from build123d import *

# Parameters (mm, degrees)
F0_R     = 18.85
F0_R_2   = 3.625
F1_DEPTH = 8
F2_SIZE  = 2
F3_T     = -1.5


with BuildPart() as f1:
    # F0 (on Top) → F1 (new body)
    with BuildSketch(Plane.XY):
        Circle(F0_R)
        Circle(F0_R_2, mode=Mode.SUBTRACT)
    extrude(amount=F1_DEPTH)

    # F2
    f2_edges = [f1.edges().sort_by_distance(p)[0] for p in [
        (-18.85, 0, 8),
    ]]
    chamfer(f2_edges, length=F2_SIZE)

    # F3
    f3_openings = [f1.faces().sort_by_distance(p)[0] for p in [
        (-18.316841, 0, 0),
    ]]
    offset(amount=F3_T, openings=f3_openings)


solid = f1.part
Input: part model. Units: mm. Frame: model coordinates. A direction names the side the tool comes from. Round coordinates to 2 decimals unless told otherwise and drop trailing zeros. Loops run counter-clockwise (first coordinate to the right, second up) from the corner with the lowest first, then second, coordinate; pieces in that order, holes last. Notation, with made-up numbers: M -17.5,74.5 L -6.5,74.5 A35 cw -6.5,111.5 Z; hole C 61,-4.5 d4. An arc over 180 degrees is marked long. Answer as CSV lines item,"result". Start each with the question number.
(1) First-contact query: pin 1 (8 mm diameter, centred on x = -7, y = 11, fed in from -Z); pin 2 (1.5 mm diameter, centred on x = -10.5, z = 7, fed in from +Y); pin 3 (3 mm diameter, centred on x = -8.5, z = 6, fed in from -Y). Flat tips, straight axial feed; report the tip coordinate or a pass-through.
(2) Draft query along Y for faces 1 (the flat face through (2.2, -3.3, 0)), 2 (the cylindrical face through (-1.111, -5.003, 3.204)), 3 (the cylindrical face through (-4.1, -18.4, 3)). Return one class per face: released by +Y, released by -Y, zero draft, split by the parting line, or undercut.
(3) Reachability of faces 4 (the flat face through (17, -5, 0)), 5 (the flat face through (-4, 4, 6.5)) from +Z, -Z, +X, -X, +Y, -Y: full face, straight path, thin tool, end or side. Return the list, or none.
(4) Section A-A, the plane y = 0. Output: boundary loops of the cut face in (x, z) (3 decimals), plus the area to 3 significant figures.
(5) Section C-C, the plane z = 2.25. Output: boundary loops of the cut face in (x, y) (3 decimals), plus the area to 3 significant figures.
(6) Line query: line 1 (Y direction, x = 0, z = 2) (3 decimals); line 2 (Z direction, x = 13, y = 1.5); line 3 (Y direction, x = 0, z = 5.75) (3 decimals). Output: solid intervals per line, ascending. Write a range as [from, to].
Values found:
1,pin 1,"stops at z = 5.69"
1,pin 2,"stops at y = 15.48"
1,pin 3,"stops at y = -17.5"
2,face 1,"zero draft"
2,face 2,"undercut"
2,face 3,"split by the parting line"
3,face 4,"-Z, +X, -X, +Y, -Y"
3,face 5,"-Z"
4,outline,"M -18.85,0 L -17.35,0 L -17.35,5.379 L -16.229,6.5 L -5.125,6.5 L -5.125,0 L -3.625,0 L -3.625,8 L -16.85,8 L -18.85,6 Z; M 3.625,0 L 5.125,0 L 5.125,6.5 L 16.229,6.5 L 17.35,5.379 L 17.35,0 L 18.85,0 L 18.85,6 L 16.85,8 L 3.625,8 Z"
4,area,"81.9 mm²"
5,outline,"C 0,0 d37.7; C 0,0 d10.25; hole C 0,0 d34.7; hole C 0,0 d7.25"
5,area,"212 mm²"
6,line 1,"y = [-18.85, -17.35], [-5.125, -3.625], [3.625, 5.125], [17.35, 18.85]"
6,line 2,"z = [6.5, 8]"
6,line 3,"y = [-18.85, -16.979], [-5.125, -3.625], [3.625, 5.125], [16.979, 18.85]"
